Model file for the job. Use its own axes, mm. Face numbers are marked on the shaded views. A direction names the side the tool comes from. Coordinates: 2 decimals unless noted, no trailing zeros. Write each loop counter-clockwise with the first axis right and the second up, starting at its lowest first coordinate (ties: lowest second). Pieces come first, ordered by that corner, then holes. Notation, with made-up numbers: (79, -7.75) - (94, -7.75) arc R18 cw to (94, 5.25) - close; hole circle Ø3 at (36, -28.5). An arc over 180 degrees is marked (long way). Put each result on its own line as item: value. Start each with the question number.
1. Drop flat-ended pins along their axis: P1, Ø7, axis at x = -3, y = 26, coming from the -Z side; P2, Ø4, axis at x = -3.5, y = 25.5, coming from the +Z side; P3, Ø1.5, axis at x = 7, y = 50, coming from the -Z side; P4, Ø9, axis at x = 0, y = 57.5, coming from the -Z side. Give the stop position or say it passes through.
2. Saw through at A-A, the plane x = 0. Write the cut outline in (y, z), plus the area to 3 significant figures.
3. Saw through at B-B, the plane y = 57.5. Write the cut outline in (x, z), plus the area to 3 significant figures.
4. Drill centre lines: L1, parallel to Y at x = 0, z = 2.75; L2, parallel to X at y = 57.5, z = 8.25; L3, parallel to Y at x = 0, z = 8.25. Where is each one in solid material? Low to high. Write a range as from..to.
5. Saw through at C-C, the plane z = 4.5. Write the cut outline in (x, y), plus the area to 3 significant figures.
6. Saw through at D-D, the plane z = 1.25. Write the cut outline in (x, y), plus the area to 3 significant figures.
7. Which spindle directions (+Z, -Z, +X, -X, +Y, -Y) get a long thin tool onto all of the face, cutting with end or side? Do the marked faces 1, 2, 3, 4 and 5. Say none if no direction does.
```python
from build123d import *

# Parameters (mm, degrees)
SKETCH1_R                       = 7.15
SKETCH1_R_2                     = 5.05
BOSS_EXTRUDE1_DEPTH             = 12.6
BOSS_EXTRUDE2_DEPTH             = 2.75
BOSS_EXTRUDE2_DEPTH_BACK        = 2.75
SKETCH2_R                       = 7.2
SKETCH2_R_2                     = 7.15
BOSS_EXTRUDE3_REACH             = 73.164
SKETCH3_R                       = 7.248211447
SKETCH3_R_2                     = 5.05
BOSS_EXTRUDE3_DIRECTION_2_REACH = 73.164


with BuildPart() as part:
    # Sketch1 → Boss-Extrude1 (new body)
    with BuildSketch(Plane.XY):
        Circle(SKETCH1_R)
        Circle(SKETCH1_R_2, mode=Mode.SUBTRACT)
    extrude(amount=BOSS_EXTRUDE1_DEPTH)

    # Sketch2 → Boss-Extrude2 (add, two sides: drawn at the far end of the back side and taken through both)
    with BuildSketch(Plane(origin=(0, 0, 6.3), x_dir=(-1, 0, 0), z_dir=(0, 0, -1)).offset(-BOSS_EXTRUDE2_DEPTH_BACK)):
        with BuildLine():
            Line((3.05, 15.617298102), (3.05, 41.882701898))
            ThreePointArc((3.05, 41.882701898), (3.851449168, 44.878543892), (6.041689751, 47.074047528))
            ThreePointArc((6.041689751, 47.074047528), (0, 69.55), (-6.041689751, 47.074047528))
            ThreePointArc((-6.041689751, 47.074047528), (-3.851449168, 44.878543892), (-3.05, 41.882701898))
            Line((-3.05, 41.882701898), (-3.05, 15.617298102))
            ThreePointArc((-3.05, 15.617298102), (-3.851449168, 12.621456108), (-6.041689751, 10.425952472))
            ThreePointArc((-6.041689751, 10.425952472), (0, -12.05), (6.041689751, 10.425952472))
            ThreePointArc((6.041689751, 10.425952472), (3.851449168, 12.621456108), (3.05, 15.617298102))
        make_face()
        with Locations((0, 57.5)):
            Circle(SKETCH2_R, mode=Mode.SUBTRACT)
        with Locations(Location((0, 0, 0), (0, 0, 180))):
            Circle(SKETCH2_R_2, mode=Mode.SUBTRACT)
    extrude(amount=BOSS_EXTRUDE2_DEPTH + BOSS_EXTRUDE2_DEPTH_BACK)

    # Boss-Extrude3: up to this face of the body (flat: up to its plane)
    boss_extrude3_end = Plane(part.part.faces().sort_by_distance((-6.947767461, 0, 0))[0])
    # Sketch3 → Boss-Extrude3 (add, up to the picked face)
    with BuildSketch(Plane(origin=(0, 0, 3.55), x_dir=(-1, 0, 0), z_dir=(0, 0, -1)), mode=Mode.PRIVATE) as boss_extrude3_sk1:
        with Locations(Location((0, 57.5, 0), (0, 0, 180))):
            Circle(SKETCH3_R)
        with Locations(Location((0, 57.5, 0), (0, 0, 180))):
            Circle(SKETCH3_R_2, mode=Mode.SUBTRACT)
    boss_extrude3_tool1 = split(extrude(boss_extrude3_sk1.sketch, amount=BOSS_EXTRUDE3_REACH, mode=Mode.PRIVATE), bisect_by=boss_extrude3_end, keep=Keep.BOTH, mode=Mode.PRIVATE)
    add(boss_extrude3_tool1.solids().sort_by(Axis((-7.043201, 57.5, 3.55), (0, 0, -1)))[0])

    # Boss-Extrude3 direction 2: up to this face of the body (flat: up to its plane)
    boss_extrude3_direction_2_end = Plane(part.part.faces().sort_by_distance((-6.947767461, 0, 12.6))[0])
    # Sketch3 → Boss-Extrude3 direction 2 (add, up to the picked face)
    with BuildSketch(Plane(origin=(0, 0, 3.55), x_dir=(-1, 0, 0), z_dir=(0, 0, -1)), mode=Mode.PRIVATE) as boss_extrude3_direction_2_sk1:
        with Locations(Location((0, 57.5, 0), (0, 0, 180))):
            Circle(SKETCH3_R)
        with Locations(Location((0, 57.5, 0), (0, 0, 180))):
            Circle(SKETCH3_R_2, mode=Mode.SUBTRACT)
    boss_extrude3_direction_2_tool1 = split(extrude(boss_extrude3_direction_2_sk1.sketch, amount=-BOSS_EXTRUDE3_DIRECTION_2_REACH, mode=Mode.PRIVATE), bisect_by=boss_extrude3_direction_2_end, keep=Keep.BOTH, mode=Mode.PRIVATE)
    add(boss_extrude3_direction_2_tool1.solids().sort_by(Axis((-7.043201, 57.5, 3.55), (0, 0, 1)))[0])


solid = part.part
```
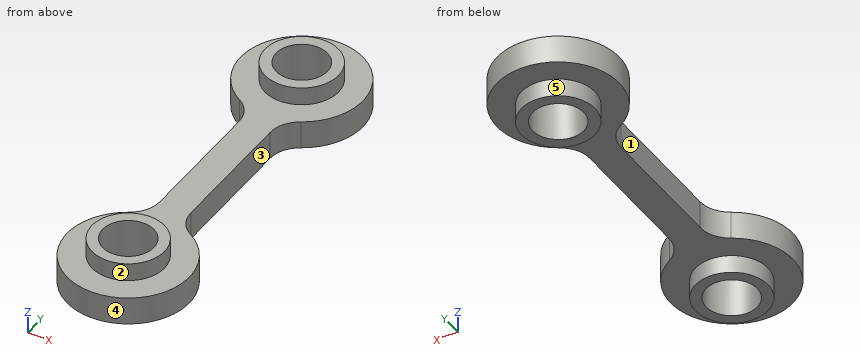
Final values:
1. P1: stops at z = 3.55
1. P2: stops at z = 9.05
1. P3: stops at z = 3.55
1. P4: passes through
2. outline: (-12.05, 3.55) - (-7.15, 3.55) - (-7.15, 0) - (-5.05, 0) - (-5.05, 12.6) - (-7.15, 12.6) - (-7.15, 9.05) - (-12.05, 9.05) - close; (5.05, 0) - (7.15, 0) - (7.15, 3.55) - (50.25, 3.55) - (50.25, 0) - (52.45, 0) - (52.45, 12.6) - (50.25, 12.6) - (50.25, 9.05) - (7.15, 9.05) - (7.15, 12.6) - (5.05, 12.6) - close; (62.55, 0) - (64.75, 0) - (64.75, 3.55) - (69.55, 3.55) - (69.55, 9.05) - (64.75, 9.05) - (64.75, 12.6) - (62.55, 12.6) - close
2. area: 399 mm²
3. outline: (-12.05, 3.55) - (-7.25, 3.55) - (-7.25, 0) - (-5.05, 0) - (-5.05, 12.6) - (-7.25, 12.6) - (-7.25, 9.05) - (-12.05, 9.05) - close; (5.05, 0) - (7.25, 0) - (7.25, 3.55) - (12.05, 3.55) - (12.05, 9.05) - (7.25, 9.05) - (7.25, 12.6) - (5.05, 12.6) - close
3. area: 108 mm²
4. L1: y = -7.15..-5.05, 5.05..7.15, 50.25..52.45, 62.55..64.75
4. L2: x = -12.05..-5.05, 5.05..12.05
4. L3: y = -12.05..-5.05, 5.05..52.45, 62.55..69.55
5. outline: (-6.04, 10.43) arc R12.05 ccw (long way) to (6.04, 10.43) arc R6 cw to (3.05, 15.62) - (3.05, 41.88) arc R6 cw to (6.04, 47.07) arc R12.05 ccw (long way) to (-6.04, 47.07) arc R6 cw to (-3.05, 41.88) - (-3.05, 15.62) arc R6 cw to start; hole circle Ø10.1 at (0, 0); hole circle Ø10.1 at (0, 57.5)
5. area: 967 mm²
6. outline: circle Ø14.5 at (0, 57.5); circle Ø14.3 at (0, 0); hole circle Ø10.1 at (0, 0); hole circle Ø10.1 at (0, 57.5)
6. area: 165 mm²
7. face 1: +Z, -Z, -X
7. face 2: +Z
7. face 3: +Z, -Z, +X
7. face 4: +Z, -Z
7. face 5: -Z
